Geometry: final body of the model. Coordinates: model frame, mm. Face numbers are marked on the shaded views. Round coordinates to 2 decimals unless told otherwise and drop trailing zeros. Order: outer loops, then holes, each group sorted by start corner. A loop starts at its lowest first (then second) coordinate and runs counter-clockwise, first axis right, second up. Notation, with made-up numbers: (-24, 75.25) - (29, 75.25) arc R21 ccw to (29, 83.25) - close; hole circle Ø5 at (-21, -30.5). An arc over 180 degrees is marked (long way). Put each result on its own line as item: value. Start each with the question number.
(1) Pull-direction query (Z, two-part tool) for the marked faces 1, 2 and 3; classes: released by +Z, released by -Z, zero draft, split by the parting line, or undercut.
(2) Pin query (flat end, axial travel): P1, Ø4.5, axis at x = 5.5, y = -174, coming from the +Z side; P2, Ø1.8, axis at y = -238.85, z = -112.86, coming from the +X side; P3, Ø1, axis at x = 8, z = -22.5, coming from the +Y side; P4, Ø1.6, axis at x = 5, z = -30.5, coming from the +Y side (3 decimals). Return the tip coordinate at first contact, or that it passes through.
(3) Material intervals for L1, parallel to Z at x = 5.5, y = -158.5; L2, parallel to Z at x = 7.75, y = -143.5; L3, parallel to Z at x = 8.75, y = -172.5, sorted ascending. Write a range as [from, to].
(4) Section A-A (y = -173). Output: boundary loops of the cut face in (x, z), and give its area (3 significant figures).
(5) Section D-D (y = -218). Output: boundary loops of the cut face in (x, z), and give its area (3 significant figures).
(6) Section C-C (y = -135.5). Output: boundary loops of the cut face in (x, z), and give its area (3 significant figures).
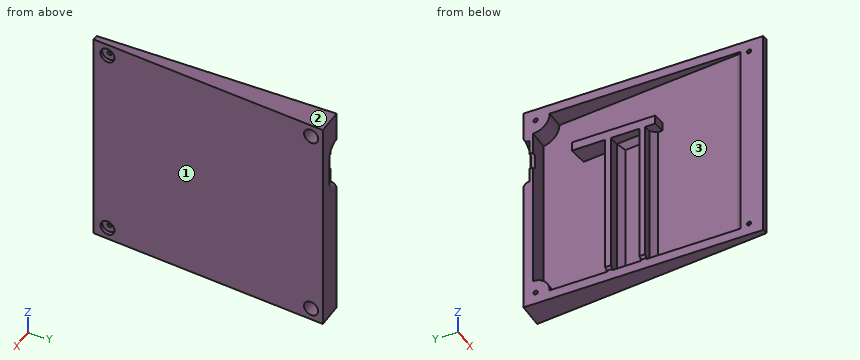
from build123d import *

# Parameters (mm, degrees)
BOSS_EXTRUDE1_DEPTH       = 119.57
CUT_EXTRUDE1_START        = -114.274828565
CUT_EXTRUDE1_DEPTH        = 109.036999581
BOSS_EXTRUDE2_OUTLINE_R   = 1.15
BOSS_EXTRUDE2_DEPTH       = 12
BOSS_EXTRUDE2_2_OUTLINE_W = 8
BOSS_EXTRUDE2_2_OUTLINE_H = 109.036999581
BOSS_EXTRUDE2_2_OUTLINE_R = 1.15
BOSS_EXTRUDE2_2_DEPTH     = 1.246713455
BOSS_EXTRUDE4_START       = -114.274828565
BOSS_EXTRUDE4_DEPTH       = 85.567402499
BOSS_EXTRUDE4_START_2     = -33.707426066
BOSS_EXTRUDE4_2_DEPTH     = 5
CHAMFER6_SIZE             = 2
CHAMFER7_SIZE             = 3
CHAMFER8_SIZE             = 3
SKETCH10_R                = 1.15
CUT_EXTRUDE2_DEPTH        = 40
CUT_EXTRUDE5_START        = -2
SKETCH11_R                = 4
CUT_EXTRUDE5_DEPTH        = 29
CUT_EXTRUDE6_START        = -1.5
SKETCH14_R                = 4
CUT_EXTRUDE6_DEPTH        = 29
CUT_EXTRUDE8_DEPTH        = 21
CUT_EXTRUDE9_DEPTH        = 3.2
FILLET2_SIZE              = 3
CUT_EXTRUDE11_REACH       = 276.65
SKETCH17_W                = 2
SKETCH17_H                = 109.036999581


with BuildPart() as part:
    # Sketch1 → Boss-Extrude1 (new body)
    with BuildSketch(Plane.XY):
        Polygon((3, -246.574899039), (5.988584094, -246.836366267), (17.398099188, -116.425012), (3, -116.425012), align=None)
    extrude(amount=-BOSS_EXTRUDE1_DEPTH)

    # Cut-Extrude1: read off the stored shape, not the designer's step
    # Cut-Extrude1 outline → Cut-Extrude1 (cut)
    with BuildSketch(Plane.XY.offset(CUT_EXTRUDE1_START)):
        Polygon((3, -240.324899039), (3.546804147, -240.324899039), (13.928199078, -121.665012), (3, -121.665012), align=None)
    extrude(amount=CUT_EXTRUDE1_DEPTH, mode=Mode.SUBTRACT)

    # Boss-Extrude2: read off the stored shape, not the designer's step
    # Boss-Extrude2 outline → Boss-Extrude2 (add)
    # profile 1 of 2: a face of its own
    with BuildSketch(Plane.YZ.offset(3)):
        with BuildLine():
            ThreePointArc((-121.665012, -105.274828565), (-128.028973031, -107.910867534), (-130.665012, -114.274828565))
            Line((-130.665012, -114.274828565), (-121.665012, -114.274828565))
            Line((-121.665012, -114.274828565), (-121.665012, -105.274828565))
        make_face()
        with Locations((-123.097401734, -112.861435085)):
            Circle(BOSS_EXTRUDE2_OUTLINE_R, mode=Mode.SUBTRACT)
    # profile 2 of 2: a face of its own
    with BuildSketch(Plane.YZ.offset(3)):
        with BuildLine():
            ThreePointArc((-130.665012, -5.237828984), (-128.02897303, -11.601790014), (-121.665012, -14.237828984))
            Line((-121.665012, -14.237828984), (-121.665012, -5.237828984))
            Line((-121.665012, -5.237828984), (-130.665012, -5.237828984))
        make_face()
        with Locations((-123.076755271, -6.637532276)):
            Circle(BOSS_EXTRUDE2_OUTLINE_R, mode=Mode.SUBTRACT)
    extrude(amount=BOSS_EXTRUDE2_DEPTH)

    # Boss-Extrude2 2 outline → Boss-Extrude2 2 (add)
    with BuildSketch(Plane.YZ.offset(3)):
        with Locations((-236.324899039, -59.756328775)):
            Rectangle(BOSS_EXTRUDE2_2_OUTLINE_W, BOSS_EXTRUDE2_2_OUTLINE_H)
        with Locations((-238.852206599, -112.861435085)):
            Circle(BOSS_EXTRUDE2_2_OUTLINE_R, mode=Mode.SUBTRACT)
        with Locations((-238.852206599, -6.631689226)):
            Circle(BOSS_EXTRUDE2_2_OUTLINE_R, mode=Mode.SUBTRACT)
    extrude(amount=BOSS_EXTRUDE2_2_DEPTH)

    # Boss-Extrude4: read off the stored shape, not the designer's step
    # Boss-Extrude4 outline → Boss-Extrude4 (add)
    with BuildSketch(Plane.XY.offset(BOSS_EXTRUDE4_START)):
        Polygon((10.373859962, -162.291294), (1.63, -161.526305378), (1.63, -164.53776489), (10.112392734, -165.279878094), align=None)
        Polygon((8.762077136, -180.714056005), (1.63, -180.090080109), (1.63, -183.101539621), (8.500609907, -183.7026401), align=None)
    extrude(amount=BOSS_EXTRUDE4_DEPTH)

    # Boss-Extrude4 2 outline → Boss-Extrude4 2 (add)
    with BuildSketch(Plane.XY.offset(BOSS_EXTRUDE4_START_2)):
        Polygon((11.942877213, -144.35734476), (1.63, -143.455084916), (1.63, -161.526305378), (10.373859962, -162.291294), align=None)
        Polygon((10.112392734, -165.279878094), (1.63, -164.53776489), (1.63, -180.090080109), (8.762077136, -180.714056005), align=None)
        Polygon((8.500609907, -183.7026401), (1.63, -183.101539621), (1.63, -188.626977605), (8.020868789, -189.186106174), align=None)
    extrude(amount=BOSS_EXTRUDE4_2_DEPTH)

    # Chamfer6
    # the kernel refuses this chamfer: 2 mm, written as the material it takes off along each edge
    with BuildSketch(Plane(origin=(1.63, -174.946714133, -114.274828565), x_dir=(0, 0, 1), z_dir=(0, -1, 0))) as chamfer6_piece_1_section:
        Polygon((CHAMFER6_SIZE, 0), (0, -CHAMFER6_SIZE), (0, 0), align=None)
    chamfer6_piece_1 = extrude(amount=13.298191464, mode=Mode.PRIVATE)
    chamfer6_piece_1 = split(chamfer6_piece_1, bisect_by=Plane(origin=(3, -174.946714133, -114.274828565), z_dir=(-1, 0, 0)), keep=Keep.TOP, mode=Mode.PRIVATE)
    add(chamfer6_piece_1, mode=Mode.SUBTRACT)
    with BuildSketch(Plane(origin=(1.63, -156.382939402, -114.274828565), x_dir=(0, 0, 1), z_dir=(0, -1, 0))) as chamfer6_piece_2_section:
        Polygon((CHAMFER6_SIZE, 0), (0, -CHAMFER6_SIZE), (0, 0), align=None)
    chamfer6_piece_2 = extrude(amount=13.298191464, mode=Mode.PRIVATE)
    chamfer6_piece_2 = split(chamfer6_piece_2, bisect_by=Plane(origin=(3, -156.382939402, -114.274828565), z_dir=(-1, 0, 0)), keep=Keep.TOP, mode=Mode.PRIVATE)
    add(chamfer6_piece_2, mode=Mode.SUBTRACT)

    # Chamfer7
    chamfer7_edges = [part.edges().sort_by_distance(p)[0] for p in [
        (10.112392734, -165.279878094, -73.991127315),
        (8.762077136, -180.714056005, -73.991127315),
        (9.437234935, -172.99696705, -33.707426066),
        (9.437234935, -172.996967049, -114.274828565),
    ]]
    chamfer(chamfer7_edges, length=CHAMFER7_SIZE)

    # Chamfer8
    chamfer8_edges = [part.edges().sort_by_distance(p)[0] for p in [
        (8.500609907, -183.7026401, -73.991127315),
        (10.373859962, -162.291294, -73.991127315),
    ]]
    chamfer(chamfer8_edges, length=CHAMFER8_SIZE)

    # Sketch10 → Cut-Extrude2 (cut)
    with BuildSketch(Plane(origin=(3, 0, 0), x_dir=(0, -1, 0), z_dir=(-1, 0, 0))):
        with Locations((123.097401734, -112.861435085)):
            Circle(SKETCH10_R)
        with Locations((123.076755271, -6.637532276)):
            Circle(SKETCH10_R)
        with Locations((238.852206599, -6.631689226)):
            Circle(SKETCH10_R)
        with Locations((238.852206599, -112.861435085)):
            Circle(SKETCH10_R)
    extrude(amount=-CUT_EXTRUDE2_DEPTH, mode=Mode.SUBTRACT)

    # Sketch11 → Cut-Extrude5 (cut)
    with BuildSketch(Plane(origin=(3, 0, 0), x_dir=(0, -1, 0), z_dir=(-1, 0, 0)).offset(CUT_EXTRUDE5_START)):
        with Locations((123.097401734, -112.861435085)):
            Circle(SKETCH11_R)
        with Locations((123.076755271, -6.637532276)):
            Circle(SKETCH11_R)
    extrude(amount=-CUT_EXTRUDE5_DEPTH, mode=Mode.SUBTRACT)

    # Sketch14 → Cut-Extrude6 (cut)
    with BuildSketch(Plane(origin=(3, 0, 0), x_dir=(0, -1, 0), z_dir=(-1, 0, 0)).offset(CUT_EXTRUDE6_START)):
        with Locations((238.852206599, -6.631689226)):
            Circle(SKETCH14_R)
        with Locations((238.852206599, -112.861435085)):
            Circle(SKETCH14_R)
    extrude(amount=-CUT_EXTRUDE6_DEPTH, mode=Mode.SUBTRACT)

    # Sketch15 → Cut-Extrude8 (cut)
    with BuildSketch(Plane(origin=(0, -116.425012, 0), x_dir=(-1, 0, 0), z_dir=(0, 1, 0))):
        with BuildLine():
            Line((-3.623758546, -26.015341992), (-2.783758546, -26.015341992))
            ThreePointArc((-2.783758546, -26.015341992), (-1.864519731, -26.396103177), (-1.483758546, -27.315341992))
            Line((-1.483758546, -27.315341992), (-1.483758546, -33.915341992))
            ThreePointArc((-1.483758546, -33.915341992), (-1.864519731, -34.834580808), (-2.783758546, -35.215341992))
            Line((-2.783758546, -35.215341992), (-3.623758546, -35.215341992))
            ThreePointArc((-3.623758546, -35.215341992), (-4.542997362, -34.834580808), (-4.923758546, -33.915341992))
            Line((-4.923758546, -33.915341992), (-4.923758546, -27.315341992))
            ThreePointArc((-4.923758546, -27.315341992), (-4.542997362, -26.396103177), (-3.623758546, -26.015341992))
        make_face()
    extrude(amount=-CUT_EXTRUDE8_DEPTH, mode=Mode.SUBTRACT)

    # Sketch16 → Cut-Extrude9 (cut)
    with BuildSketch(Plane(origin=(0, -116.425012, 0), x_dir=(-1, 0, 0), z_dir=(0, 1, 0))):
        with BuildLine():
            Line((-8.203758546, -38.115341992), (-8.203758546, -23.115341992))
            ThreePointArc((-8.203758546, -23.115341992), (-3.203758546, -18.115341992), (1.796241454, -23.115341992))
            Line((1.796241454, -23.115341992), (1.796241454, -38.115341992))
            ThreePointArc((1.796241454, -38.115341992), (-3.203758546, -43.115341992), (-8.203758546, -38.115341992))
        make_face()
    extrude(amount=-CUT_EXTRUDE9_DEPTH, mode=Mode.SUBTRACT)

    # Fillet2
    # a fillet whose section is not a circle: 3 mm, written as the material it takes off along each edge
    with BuildSketch(Plane(origin=(3.203758546, -116.425012, -23.115341992), x_dir=(1, 0, 0), z_dir=(0, 0, -1))) as fillet2_piece_1:
        with BuildLine():
            Bezier((5 + FILLET2_SIZE, 0), (5, 0), (5, FILLET2_SIZE), weights=[1, 0.707106781, 1])
            Line((5, FILLET2_SIZE), (5, 0))
            Line((5, 0), (5 + FILLET2_SIZE, 0))
        make_face()
    revolve(axis=Axis((3.203758546, -116.425012, -23.115341992), (0, -1, 0)), revolution_arc=178.315556871, mode=Mode.SUBTRACT)
    with BuildSketch(Plane(origin=(8.203758546, -116.425012, -38.115341992), x_dir=(1, 0, 0), z_dir=(0, 0, 1))) as fillet2_piece_2:
        with BuildLine():
            Bezier((FILLET2_SIZE, 0), (0, 0), (0, -FILLET2_SIZE), weights=[1, 0.707106781, 1])
            Line((0, -FILLET2_SIZE), (0, 0))
            Line((0, 0), (FILLET2_SIZE, 0))
        make_face()
    extrude(amount=15, mode=Mode.SUBTRACT)
    with BuildSketch(Plane(origin=(3.203758546, -116.425012, -38.115341992), x_dir=(-0.9995678782122136, 0, -0.02939484387325848), z_dir=(-0.02939484387325848, 0, 0.9995678782122136))) as fillet2_piece_3:
        with BuildLine():
            Bezier((5 + FILLET2_SIZE, 0), (5, 0), (5, FILLET2_SIZE), weights=[1, 0.707106781, 1])
            Line((5, FILLET2_SIZE), (5, 0))
            Line((5, 0), (5 + FILLET2_SIZE, 0))
        make_face()
    revolve(axis=Axis((3.203758546, -116.425012, -38.115341992), (0, -1, 0)), revolution_arc=178.315556871, mode=Mode.SUBTRACT)

    # Cut-Extrude11: up to this plane
    cut_extrude11_end = Plane(origin=(2.988584094, -246.836366267, -119.57), z_dir=(0.9961946980917459, -0.08715574274765435, 0))
    # Sketch17 → Cut-Extrude11 (cut, up to the surface)
    with BuildSketch(Plane(origin=(3, 0, 0), x_dir=(0, -1, 0), z_dir=(-1, 0, 0)), mode=Mode.PRIVATE) as cut_extrude11_sk1:
        with Locations((233.324899039, -59.756328775)):
            Rectangle(SKETCH17_W, SKETCH17_H)
    cut_extrude11_tool1 = split(extrude(cut_extrude11_sk1.sketch, amount=-CUT_EXTRUDE11_REACH, mode=Mode.PRIVATE), bisect_by=cut_extrude11_end, keep=Keep.BOTH, mode=Mode.PRIVATE)
    add(cut_extrude11_tool1.solids().sort_by_distance((3, -233.324899, -59.756329))[0], mode=Mode.SUBTRACT)


solid = part.part
Checks:
1. face 1: zero draft
1. face 2: released by +Z
1. face 3: undercut
2. P1: stops at z = 0
2. P2: passes through
2. P3: stops at y = -118.05
2. P4: stops at y = -119.625
3. L1: z = [-119.57, -114.27], [-33.71, -28.71], [-5.24, 0]
3. L2: z = [-119.57, -114.27], [-5.24, 0]
3. L3: z = [-119.57, -112], [-35.98, -28.71], [-5.24, 0]
4. outline: (1.63, -33.71) - (6.43, -33.71) - (9.44, -36.71) - (9.44, -111.27) - (6.43, -114.27) - (3, -114.27) - (3, -119.57) - (12.45, -119.57) - (12.45, 0) - (3, 0) - (3, -5.24) - (9.44, -5.24) - (9.44, -28.71) - (1.63, -28.71) - close
4. area: 476 mm²
5. outline: (3, -119.57) - (8.51, -119.57) - (8.51, 0) - (3, 0) - (3, -5.24) - (5.5, -5.24) - (5.5, -114.27) - (3, -114.27) - close
5. area: 386 mm²
6. outline: (3, -119.57) - (15.73, -119.57) - (15.73, 0) - (3, 0) - (3, -5.24) - (12.72, -5.24) - (12.72, -114.27) - (3, -114.27) - close
6. area: 462 mm²
